Geometry: final body of the model. Coordinates: model frame, mm. Face numbers are marked on the shaded views. Give positions to 0.01 mm unless a question says otherwise; leave off trailing zeros. Write each loop counter-clockwise with the first axis right and the second up, starting at its lowest first coordinate (ties: lowest second). Pieces come first, ordered by that corner, then holes.
Q1. Cut plane C-C on x = -85. Return the cut outline in (y, z), plus the area to 3 significant figures.
Q2. Cut plane B-B on x = 66.5. Return the cut outline in (y, z).
Q3. Cut plane A-A on y = 35. Return the cut outline in (x, z), plus the area to 3 significant figures.
Q4. Pin query (flat end, axial travel): pin 1 (1.8 mm diameter, centred on x = 81.5, z = -1.5, fed in from -Y); pin 2 (5 mm diameter, centred on x = 51.5, y = -48, fed in from -Z); pin 3 (5 mm diameter, centred on y = -56, z = -4.5, fed in from +X). Return the tip coordinate at first contact, or that it passes through.
Q5. Line query: L1, parallel to X at y = -56.5, z = -4; L2, parallel to X at y = -25.5, z = 1; L3, parallel to Z at x = 71.5, y = 48. Output: solid intervals per line, ascending.
Q6. Draft query along X for the marked faces 1 and 2. Return one class per face: pulls with the +X half, pulls with the -X half, needs draft (parallel to the pull), parting line crosses it, or undercut.
```python
from build123d import *

# Parameters (mm, degrees)
F0_W       = 206
F0_H       = 138
F0_W_2     = 156
F0_H_2     = 88
F1_DEPTH   = 1.5
F2_W       = 10
F2_H       = 10
F2_R       = 1.55
F3_DEPTH   = 6
F4_DEPTH   = 9
F5_SIZE2   = 2
F5_SIZE    = 1
F5_2_SIZE2 = 2
F5_2_SIZE  = 1
F5_3_SIZE2 = 2
F5_3_SIZE  = 1
F5_4_SIZE2 = 2
F5_4_SIZE  = 1


with BuildPart() as f1:
    # F0 (on Top) → F1 (new body)
    with BuildSketch(Plane.XY):
        Rectangle(F0_W, F0_H)
        Rectangle(F0_W_2, F0_H_2, mode=Mode.SUBTRACT)
    extrude(amount=F1_DEPTH)

    # F2 (on face) → F3 (join)
    with BuildSketch(Plane(origin=(0, 0, 0), x_dir=(1, 0, 0), z_dir=(0, 0, -1))):
        with Locations((-76, 54)):
            Rectangle(F2_W, F2_H)
        with Locations((-76, 54)):
            Circle(F2_R, mode=Mode.SUBTRACT)
        with Locations((80.9, 54)):
            Rectangle(F2_W, F2_H)
        with Locations((80.9, 54)):
            Circle(F2_R, mode=Mode.SUBTRACT)
        with Locations((80.9, -60.96)):
            Rectangle(F2_W, F2_H)
        with Locations((80.9, -60.96)):
            Circle(F2_R, mode=Mode.SUBTRACT)
        with Locations((-76, -60.96)):
            Rectangle(F2_W, F2_H)
        with Locations((-76, -60.96)):
            Circle(F2_R, mode=Mode.SUBTRACT)
        with Locations((-76, 54)):
            Circle(F2_R)
        with Locations((-76, -60.96)):
            Circle(F2_R)
        with Locations((80.9, -60.96)):
            Circle(F2_R)
        with Locations((80.9, 54)):
            Circle(F2_R)
    extrude(amount=F3_DEPTH)

    # F2 (on face) → F4 (join)
    with BuildSketch(Plane(origin=(0, 0, 0), x_dir=(1, 0, 0), z_dir=(0, 0, -1))):
        with Locations((-76, 54)):
            Circle(F2_R)
        with Locations((-76, -60.96)):
            Circle(F2_R)
        with Locations((80.9, -60.96)):
            Circle(F2_R)
        with Locations((80.9, 54)):
            Circle(F2_R)
    extrude(amount=F4_DEPTH)

    # F5
    f5_edges = [f1.edges().sort_by_distance(p)[0] for p in [
        (-77.55, -54, -9),
    ]]
    f5_side = f1.faces().sort_by_distance((-76, -54, -9))[0]
    chamfer(f5_edges, length=F5_SIZE, length2=F5_SIZE2, reference=f5_side)

    # F5#2
    f5_2_edges = [f1.edges().sort_by_distance(p)[0] for p in [
        (-77.55, 60.96, -9),
    ]]
    f5_2_side = f1.faces().sort_by_distance((-76, 60.96, -9))[0]
    chamfer(f5_2_edges, length=F5_2_SIZE, length2=F5_2_SIZE2, reference=f5_2_side)

    # F5#3
    f5_3_edges = [f1.edges().sort_by_distance(p)[0] for p in [
        (79.35, -54, -9),
    ]]
    f5_3_side = f1.faces().sort_by_distance((80.9, -54, -9))[0]
    chamfer(f5_3_edges, length=F5_3_SIZE, length2=F5_3_SIZE2, reference=f5_3_side)

    # F5#4
    f5_4_edges = [f1.edges().sort_by_distance(p)[0] for p in [
        (79.35, 60.96, -9),
    ]]
    f5_4_side = f1.faces().sort_by_distance((80.9, 60.96, -9))[0]
    chamfer(f5_4_edges, length=F5_4_SIZE, length2=F5_4_SIZE2, reference=f5_4_side)


solid = f1.part
```
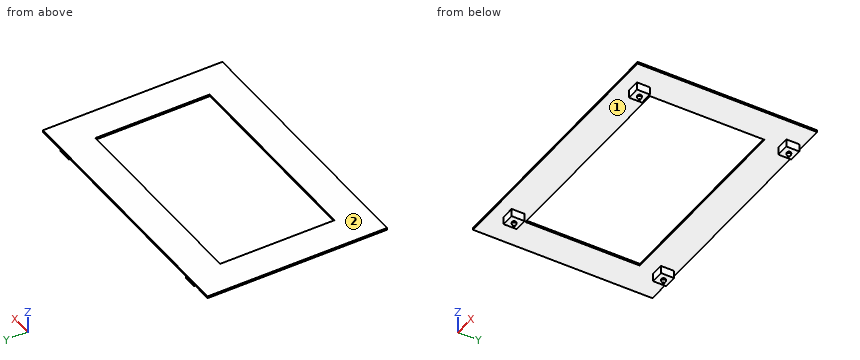
Data:
1. outline: (-69, 0) - (69, 0) - (69, 1.5) - (-69, 1.5) - close
1. area: 207 mm2
2. outline: (-69, 0) - (-44, 0) - (-44, 1.5) - (-69, 1.5) - close; (44, 0) - (69, 0) - (69, 1.5) - (44, 1.5) - close
3. outline: (-103, 0) - (-78, 0) - (-78, 1.5) - (-103, 1.5) - close; (78, 0) - (103, 0) - (103, 1.5) - (78, 1.5) - close
3. area: 75.0 mm2
4. pin 1: stops at y = -59
4. pin 2: stops at z = 0
4. pin 3: stops at x = 85.9
5. L1: x = -81 to -71, 75.9 to 85.9
5. L2: x = -103 to -78, 78 to 103
5. L3: z = 0 to 1.5
6. face 1: undercut
6. face 2: needs draft
